Geometry: final body of the model. Coordinates: model frame, mm. Round coordinates to 2 decimals unless told otherwise and drop trailing zeros. Loops run counter-clockwise (first coordinate to the right, second up) from the corner with the lowest first, then second, coordinate; pieces in that order, holes last. Notation, with made-up numbers: M -28,44.25 L 2,44.25 A18 ccw 2,53.25 Z; hole C 89,29 d6. An arc over 180 degrees is marked long. Answer as a JSON object with one key per item and string values.
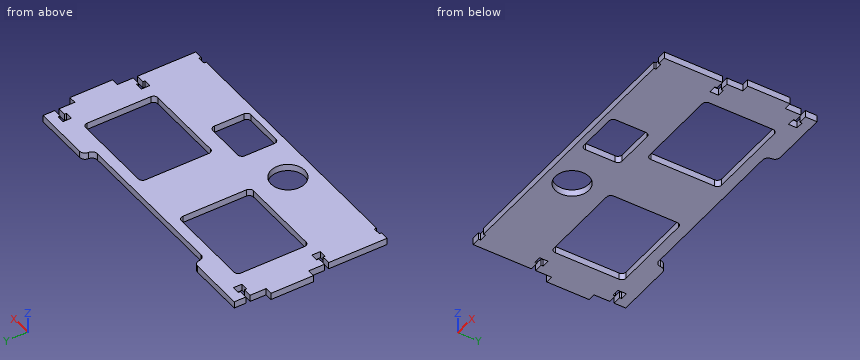
from build123d import *

# Parameters (mm, degrees)
BOSS_EXTRUDE1_DEPTH     = 3.175
CUT_EXTRUDE1_DEPTH      = 82.916607748
MIRROR2_COPY_1_DEPTH    = 82.916607748
SKETCH4_W               = 138
SKETCH4_H               = 9
BOSS_EXTRUDE3_DEPTH     = 3.175
CUT_EXTRUDE2_DEPTH      = 87.459994362
CUT_EXTRUDE2_DEPTH_BACK = 87.459994362
SKETCH5_W               = 80
SKETCH5_H               = 5
FILLET1_R               = 2.5
SKETCH6_W               = 3.5
SKETCH6_H               = 1
CUT_EXTRUDE3_DEPTH      = 87.459994362
SKETCH10_W              = 42
SKETCH10_H              = 34
CUT_EXTRUDE4_DEPTH      = 87.459994362
FILLET2_R               = 2
FILLET2_OF_MIRROR4_R    = 2
SKETCH11_R              = 7.9375
CUT_EXTRUDE5_DEPTH      = 10
SKETCH12_W              = 22
SKETCH12_H              = 18
CUT_EXTRUDE6_DEPTH      = 10
FILLET3_R               = 2


with BuildPart() as part:
    # Sketch1 → Boss-Extrude1 (new body)
    with BuildSketch(Plane.XY):
        Polygon((-69, -10), (-69, -38), (69, -38), (69, -10), (72.5, -10), (72.5, 10), (69, 10), (69, 25), (-69, 25), (-69, 10), (-72.5, 10), (-72.5, -10), align=None)
    extrude(amount=-BOSS_EXTRUDE1_DEPTH)

    # Sketch2 → Cut-Extrude1 (cut, symmetric)
    with BuildSketch(Plane.XY):
        Polygon((-69, 19.5), (-65, 19.5), (-65, 20.5), (-61.5, 20.5), (-61.5, 16.5), (-65, 16.5), (-65, 17.5), (-69, 17.5), align=None)
    cut_extrude1 = extrude(amount=CUT_EXTRUDE1_DEPTH, both=True, mode=Mode.SUBTRACT)

    # Mirror1: Cut-Extrude1 across plane
    add(cut_extrude1.mirror(Plane.ZY), mode=Mode.SUBTRACT)

    # Mirror2: Cut-Extrude1 across plane
    add(cut_extrude1.mirror(Plane.ZX), mode=Mode.SUBTRACT)

    # Mirror2 copy 1 sketch → Mirror2 copy 1 (cut, symmetric)
    with BuildSketch(Plane(origin=(0, 0, 0), x_dir=(-1, 0, 0), z_dir=(0, 0, 1))):
        Polygon((-69, 19.5), (-65, 19.5), (-65, 20.5), (-61.5, 20.5), (-61.5, 16.5), (-65, 16.5), (-65, 17.5), (-69, 17.5), align=None)
    extrude(amount=MIRROR2_COPY_1_DEPTH, both=True, mode=Mode.SUBTRACT)

    # Sketch4 → Boss-Extrude3 (add)
    with BuildSketch(Plane.XY):
        with Locations((0, -42.5)):
            Rectangle(SKETCH4_W, SKETCH4_H)
    extrude(amount=-BOSS_EXTRUDE3_DEPTH)

    # Sketch5 → Cut-Extrude2 (cut, two sides: drawn at the far end of the back side and taken through both)
    with BuildSketch(Plane.XY.offset(-CUT_EXTRUDE2_DEPTH_BACK)):
        with Locations((0, 22.5)):
            Rectangle(SKETCH5_W, SKETCH5_H)
    extrude(amount=CUT_EXTRUDE2_DEPTH + CUT_EXTRUDE2_DEPTH_BACK, mode=Mode.SUBTRACT)

    # Fillet1
    fillet1_edges = [part.edges().sort_by_distance(p)[0] for p in [
        (40, 20, -1.5875),
        (-40, 20, -1.5875),
    ]]
    fillet(fillet1_edges, radius=FILLET1_R)
    fillet1_2_edges = [part.edges().sort_by_distance(p)[0] for p in [
        (40, 25, -1.5875),
        (-40, 25, -1.5875),
    ]]
    fillet(fillet1_2_edges, radius=FILLET1_R - 0.0001)  # a hair under: the kernel refuses the full size

    # Sketch6 → Cut-Extrude3 (cut, symmetric)
    with BuildSketch(Plane.XY):
        with Locations((63.25, -46.5)):
            Rectangle(SKETCH6_W, SKETCH6_H)
    cut_extrude3 = extrude(amount=CUT_EXTRUDE3_DEPTH, both=True, mode=Mode.SUBTRACT)

    # Mirror3: Cut-Extrude3 across plane
    add(cut_extrude3.mirror(Plane.ZY), mode=Mode.SUBTRACT)

    # Sketch10 → Cut-Extrude4 (cut, through all)
    with BuildSketch(Plane(origin=(0, 0, -3.175), x_dir=(-1, 0, 0), z_dir=(0, 0, -1))):
        with Locations((34.5, -2)):
            Rectangle(SKETCH10_W, SKETCH10_H)
    cut_extrude4 = extrude(amount=-CUT_EXTRUDE4_DEPTH, mode=Mode.SUBTRACT)

    # Fillet2
    fillet2_edges = [part.edges().sort_by_distance(p)[0] for p in [
        (-55.5, 15, -1.5875),
        (-55.5, -19, -1.5875),
        (-13.5, -19, -1.5875),
        (-13.5, 15, -1.5875),
    ]]
    fillet(fillet2_edges, radius=FILLET2_R)

    # Mirror4: Cut-Extrude4 across plane
    add(cut_extrude4.mirror(Plane.ZY), mode=Mode.SUBTRACT)

    # Fillet2 of Mirror4
    fillet2_of_mirror4_edges = [part.edges().sort_by_distance(p)[0] for p in [
        (55.5, 15, -1.5875),
        (55.5, -19, -1.5875),
        (13.5, -19, -1.5875),
        (13.5, 15, -1.5875),
    ]]
    fillet(fillet2_of_mirror4_edges, radius=FILLET2_OF_MIRROR4_R)

    # Sketch11 → Cut-Extrude5 (cut)
    with BuildSketch(Plane(origin=(0, 0, -3.175), x_dir=(-1, 0, 0), z_dir=(0, 0, -1))):
        with Locations((15.875, -35)):
            Circle(SKETCH11_R)
    extrude(amount=-CUT_EXTRUDE5_DEPTH, mode=Mode.SUBTRACT)

    # Sketch12 → Cut-Extrude6 (cut)
    with BuildSketch(Plane(origin=(0, 0, -3.175), x_dir=(-1, 0, 0), z_dir=(0, 0, -1))):
        with Locations((-15.5, -35)):
            Rectangle(SKETCH12_W, SKETCH12_H)
    extrude(amount=-CUT_EXTRUDE6_DEPTH, mode=Mode.SUBTRACT)

    # Fillet3
    fillet3_edges = [part.edges().sort_by_distance(p)[0] for p in [
        (4.5, -26, -1.5875),
        (4.5, -44, -1.5875),
        (26.5, -44, -1.5875),
        (26.5, -26, -1.5875),
    ]]
    fillet(fillet3_edges, radius=FILLET3_R)


solid = part.part
1) Section query A-A (y = 4). Return the cut outline in (x, z) (3 decimals), and give its area (3 significant figures).
Results:
{"outline": "M -72.5,-3.175 L -55.5,-3.175 L -55.5,0 L -72.5,0 Z; M -13.5,-3.175 L 13.5,-3.175 L 13.5,0 L -13.5,0 Z; M 55.5,-3.175 L 72.5,-3.175 L 72.5,0 L 55.5,0 Z", "area": "194 mm2"}
2) Ray query, line 1 (X direction, y = -11, z = -0.35); line 2 (X direction, y = 0, z = -0.45); line 3 (Y direction, x = -16, z = -1.15). Return the intervals inside material, ascending.
Results:
{"line 1": "-69 to -55.5, -13.5 to 13.5, 55.5 to 69", "line 2": "-72.5 to -55.5, -13.5 to 13.5, 55.5 to 72.5", "line 3": "-47 to -42.94, -27.06 to -19, 15 to 20"}
3) Section query B-B (x = 10.5). Return the cut outline in (y, z) (3 decimals).
Results:
{"outline": "M -47,-3.175 L -44,-3.175 L -44,0 L -47,0 Z; M -26,-3.175 L 20,-3.175 L 20,0 L -26,0 Z"}
4) Section query C-C (y = -35). Return the cut outline in (x, z) (1 decimal), and give its area (3 significant figures).
Results:
{"outline": "M -69,-3.2 L -23.8,-3.2 L -23.8,0 L -69,0 Z; M -7.9,-3.2 L 4.5,-3.2 L 4.5,0 L -7.9,0 Z; M 26.5,-3.2 L 69,-3.2 L 69,0 L 26.5,0 Z", "area": "318 mm2"}
5) Pin query (flat end, axial travel): P1, Ø1.6, axis at y = 23, z = -2, coming from the -X side; P2, Ø0.5, axis at y = 17, z = -1, coming from the +X side; P3, Ø1.6, axis at x = -63.5, z = -2.5, coming from the -Y side. Return the tip coordinate at first contact, or that it passes through.
Results:
{"P1": "x = -69", "P2": "x = 69", "P3": "y = -46"}
6) Section query D-D (z = -2.3). Count the separate pieces of the cut face and the enclosed holes in it, and give its area (3 significant figures).
Results:
{"separate pieces": "1", "enclosed holes": "4", "area": "6,140 mm2"}
